The model under review builds one solid part; all positions refer to its coordinate system, in mm. Face numbers are marked on the shaded views. Round coordinates to 2 decimals unless told otherwise and drop trailing zeros. Order: outer loops, then holes, each group sorted by start corner. A loop starts at its lowest first (then second) coordinate and runs counter-clockwise, first axis right, second up.
1) To check wall thickness, follow L1, parallel to X at y = 2.5, z = -31.5; L2, parallel to X at y = 6, z = -21; L3, parallel to Y at x = 45.5, z = -20. State the ranges of each line that lie inside material, in increasing order.
2) Consider section A-A (y = 0). Give the boundary of the cut face in (x, z).
3) Clearance check with a flat-ended pin moving along its axis: P1, Ø1, axis at x = 6, y = -30.5, coming from the +Z side. State where the tip first meets the part, or that it passes through.
4) Mouldability with a two-part tool opening along X and no side actions: class the marked faces 1, 2 and 3 as pulls with the +X half, pulls with the -X half, needs draft (parallel to the pull), parting line crosses it, or undercut.
5) Consider section C-C (z = -29). Give the boundary of the cut face in (x, y).
6) Consider section B-B (x = 43.5). Give the boundary of the cut face in (y, z).
from build123d import *

# Parameters (mm, degrees)
F0_W     = 139.7
F0_H     = 116.84
F0_R     = 12.7
F1_DEPTH = 50.8


# Not quite as in the source:
# - the program builds the solid bodies; features that only make, move or delete a surface that nothing else refers to are left out


with BuildPart() as f1:
    # F0 (on Top) → F1 (new body)
    with BuildSketch(Plane.XY):
        with Locations((-10.3572173724, -0.2563824468)):
            Rectangle(F0_W, F0_H)
        with Locations((-61.2939819694, 0)):
            Circle(F0_R, mode=Mode.SUBTRACT)
        with BuildLine():
            ThreePointArc((27.8118101201, 0), (40.5118101201, 12.7), (53.2118101201, 0))
            ThreePointArc((53.2118101201, 0), (40.5118101201, -12.7), (27.8118101201, 0))
        make_face(mode=Mode.SUBTRACT)
    extrude(amount=-F1_DEPTH)


solid = f1.part
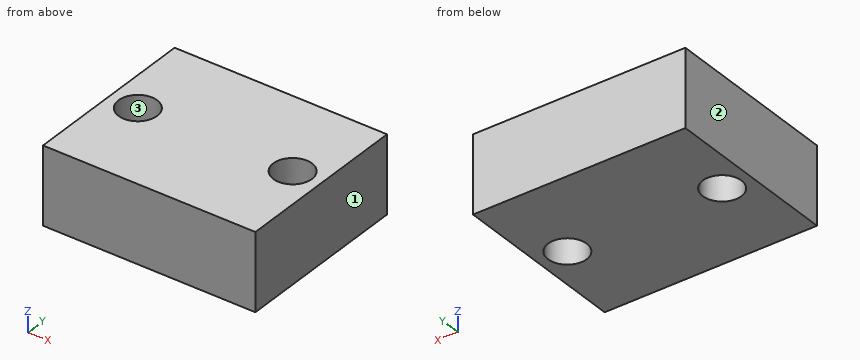
Answer below:
1. L1: x = -80.21 to -73.75, -48.84 to 28.06, 52.96 to 59.49
1. L2: x = -80.21 to -72.49, -50.1 to 29.32, 51.71 to 59.49
1. L3: y = -58.68 to -11.68, 11.68 to 58.16
2. outline: (-80.21, -50.8) - (-73.99, -50.8) - (-73.99, 0) - (-80.21, 0) - close; (-48.59, -50.8) - (27.81, -50.8) - (27.81, 0) - (-48.59, 0) - close; (53.21, -50.8) - (59.49, -50.8) - (59.49, 0) - (53.21, 0) - close
3. P1: stops at z = 0
4. face 1: pulls with the +X half
4. face 2: pulls with the -X half
4. face 3: undercut
5. outline: (-80.21, -58.68) - (59.49, -58.68) - (59.49, 58.16) - (-80.21, 58.16) - close; hole circle Ø25.4 at (-61.29, 0); hole circle Ø25.4 at (40.51, 0)
6. outline: (-58.68, -50.8) - (-12.34, -50.8) - (-12.34, 0) - (-58.68, 0) - close; (12.34, -50.8) - (58.16, -50.8) - (58.16, 0) - (12.34, 0) - close
